```python
from build123d import *

# Parameters (mm, degrees)
BOSS_EXTRUDE1_DEPTH = 24
SKETCH2_R           = 1.25
CUT_EXTRUDE1_DEPTH  = 90
CUT_EXTRUDE2_REACH  = 83.273
SKETCH3_R           = 3
SKETCH4_R           = 3
BOSS_EXTRUDE2_DEPTH = 5


with BuildPart() as part:
    # Sketch1 → Boss-Extrude1 (new body)
    with BuildSketch(Plane.XY):
        Polygon((-22.371784864, -30.407843619), (-20.871784864, -30.407843619), (-20.871784864, 9.592156381), (64.128215136, 9.592156381), (64.128215136, -30.407843619), (65.628215136, -30.407843619), (65.628215136, 11.092156381), (-22.371784864, 11.092156381), align=None)
    extrude(amount=BOSS_EXTRUDE1_DEPTH)

    # Sketch2 → Cut-Extrude1 (cut)
    with BuildSketch(Plane.ZY.offset(22.371784864)):
        with Locations((3, -22.407843619)):
            Circle(SKETCH2_R)
        with Locations((21, -22.407843619)):
            Circle(SKETCH2_R)
    extrude(amount=-CUT_EXTRUDE1_DEPTH, mode=Mode.SUBTRACT)

    # Sketch3 → Cut-Extrude2 (cut, up to next)
    with BuildSketch(Plane(origin=(0, 11.092156381, 0), x_dir=(1, 0, 0), z_dir=(0, 1, 0)), mode=Mode.PRIVATE) as cut_extrude2_sk1:
        with Locations(Location((21.628215136, -12, 0), (0, 0, 180))):
            Circle(SKETCH3_R)
    cut_extrude2_tool1 = extrude(cut_extrude2_sk1.sketch, amount=-CUT_EXTRUDE2_REACH, mode=Mode.PRIVATE) & part.part
    add(cut_extrude2_tool1.solids().sort_by_distance((21.628215, 11.092156, 12))[0], mode=Mode.SUBTRACT)

    # Sketch4 → Boss-Extrude2 (add)
    with BuildSketch(Plane.XZ.offset(-9.592156381)):
        Polygon((18.628215136, 6.803847577), (24.628215136, 6.803847577), (27.628215136, 12), (24.628215136, 17.196152423), (18.628215136, 17.196152423), (15.628215136, 12), align=None)
        with Locations(Location((21.628215136, 12, 0), (0, 0, 180))):
            Circle(SKETCH4_R, mode=Mode.SUBTRACT)
    extrude(amount=BOSS_EXTRUDE2_DEPTH)


solid = part.part
```
Build history of the part. All positions in model axes, mm. A direction names the side the tool comes from. Round coordinates to 2 decimals unless told otherwise and drop trailing zeros. Order: outer loops, then holes, each group sorted by start corner. A loop starts at its lowest first (then second) coordinate and runs counter-clockwise, first axis right, second up. Notation, with made-up numbers: (-34.75, 52) -> (22.25, 52) arc R17 ccw to (22.25, 73) -> close; hole circle Ø8 at (18.5, -1.75). An arc over 180 degrees is marked (long way). Answer in a Markdown table with one row per item.
1) Band-saw the part on D-D on z = 8. Give the cut face in (x, y).
Values:
| item | result |
|---|---|
| outline | (-22.37, -30.41) -> (-20.87, -30.41) -> (-20.87, 9.59) -> (17.94, 9.59) -> (17.94, 4.59) -> (25.32, 4.59) -> (25.32, 9.59) -> (64.13, 9.59) -> (64.13, -30.41) -> (65.63, -30.41) -> (65.63, 11.09) -> (-22.37, 11.09) -> close |
2) Band-saw the part on C-C on y = 8.5. Give the cut face in (x, z), and give its area (3 significant figures).
Values:
| item | result |
|---|---|
| outline | (-22.37, 0) -> (-20.87, 0) -> (-20.87, 24) -> (-22.37, 24) -> close; (15.63, 12) -> (18.63, 6.8) -> (24.63, 6.8) -> (27.63, 12) -> (24.63, 17.2) -> (18.63, 17.2) -> close; (64.13, 0) -> (65.63, 0) -> (65.63, 24) -> (64.13, 24) -> close; hole circle Ø6 at (21.63, 12) |
| area | 137 mm2 |
3) Which spindle directions (+Z, -Z, +X, -X, +Y, -Y) get a long thin tool onto all of the face, cutting with end or side? Do faces 4 (the flat face through (64.128, -10, 12)), 5 (the cylindrical face through (64.868, -22.887, 22.155)), 6 (the cylindrical face through (18.767, 7.888, 11.099)), 7 (the flat face through (26.11, 7.13, 9.37)), 8 (the flat face through (22, 7, 17.196)). Say none if no direction does.
Values:
| item | result |
|---|---|
| face 4 | +Z, -Z, -Y |
| face 5 | +X, -X |
| face 6 | +Y, -Y |
| face 7 | -Z, -Y |
| face 8 | +Z, -Y |
4) Pin check, flat tips, straight feed: P1, Ø7, axis at x = 21.63, z = 12, coming from the -Y side; P2, Ø1.5, axis at x = 22.5, y = 6, coming from the -Z side; P3, Ø10, axis at x = 53, z = 16.5, coming from the -Y side; P4, Ø1.5, axis at y = -22.41, z = 21, coming from the -X side. Stop position of each tip, or through.
Values:
| item | result |
|---|---|
| P1 | y = 4.59 |
| P2 | z = 6.8 |
| P3 | y = 9.59 |
| P4 | through |
5) Mould opens along X. For faces 1 (the flat face through (65.628, -10, 12)), 2 (the flat face through (17.149, 7.127, 14.634)), 3 (the cylindrical face through (-21.632, -22.887, 22.155)) say: released by +X, released by -X, zero draft, split by the parting line, or undercut.
Values:
| item | result |
|---|---|
| face 1 | released by +X |
| face 2 | undercut |
| face 3 | zero draft |
6) Wall check: L1, parallel to X at y = 8.75, z = 12; L2, parallel to X at y = -24, z = 2.25; L3, parallel to Y at x = -22, z = 3. Give the ranges that are in metal, low to high.
Values:
| item | result |
|---|---|
| L1 | -22.37 to -20.87, 15.63 to 18.63, 24.63 to 27.63, 64.13 to 65.63 |
| L2 | -22.37 to -20.87, 64.13 to 65.63 |
| L3 | -30.41 to -23.66, -21.16 to 11.09 |
7) Band-saw the part on A-A on y = -11. Give the cut face in (x, z).
Values:
| item | result |
|---|---|
| outline | (-22.37, 0) -> (-20.87, 0) -> (-20.87, 24) -> (-22.37, 24) -> close; (64.13, 0) -> (65.63, 0) -> (65.63, 24) -> (64.13, 24) -> close |
8) Band-saw the part on B-B on z = 21. Give the cut face in (x, y), and give its area (4 significant figures).
Values:
| item | result |
|---|---|
| outline | (-22.37, -30.41) -> (-20.87, -30.41) -> (-20.87, -23.66) -> (-22.37, -23.66) -> close; (-22.37, -21.16) -> (-20.87, -21.16) -> (-20.87, 9.59) -> (64.13, 9.59) -> (64.13, -21.16) -> (65.63, -21.16) -> (65.63, 11.09) -> (-22.37, 11.09) -> close; (64.13, -30.41) -> (65.63, -30.41) -> (65.63, -23.66) -> (64.13, -23.66) -> close |
| area | 244.5 mm2 |
